Geometry check sheet. Reference: the model listing, model coordinates, mm. Face numbers are marked on the shaded views. A direction names the side the tool comes from. Give positions to 0.01 mm unless a question says otherwise; leave off trailing zeros. Write each loop counter-clockwise with the first axis right and the second up, starting at its lowest first coordinate (ties: lowest second). Pieces come first, ordered by that corner, then holes.
(1) Mould release check, pull along X, two halves, no side actions. Record for the marked faces 1, 2, 3 and 4: +X half, -X half, draft (parallel to the pull), parting line (faces both ways), or undercut.
(2) Thickness scan on line 1 along X through (y, z) = (-12, 5) (3 decimals); line 2 along X through (y, z) = (-8, 14.5) (3 decimals); line 3 along Y through (x, z) = (35, 32). Record the ranges inside material, lowest first.
(3) Cross-section at A-A (y = -21). Record the boundary of the cut face in (x, z) (3 decimals).
(4) Cross-section at B-B (y = 11.5). Record the boundary of the cut face in (x, z) (3 decimals).
(5) Depth check by flat-ended pin: P1, Ø16.5, axis at x = 2, y = 47, coming from the +Z side (3 decimals); P2, Ø2.5, axis at x = 59.5, y = 0, coming from the -Z side; P3, Ø8.5, axis at y = 13, z = 20.5, coming from the -X side (3 decimals). Enter the tip coordinate at first touch or a pass-through.
(6) Cross-section at C-C (y = 38.5). Record the boundary of the cut face in (x, z) (3 decimals), and give its area (3 significant figures).
(7) Tool access check on the marked faces 5, 6 and 7. Record the directions out of +Z, -Z, +X, -X, +Y, -Y that give a thin tool (end or side, any length) a straight path to the whole face; none if there is none.
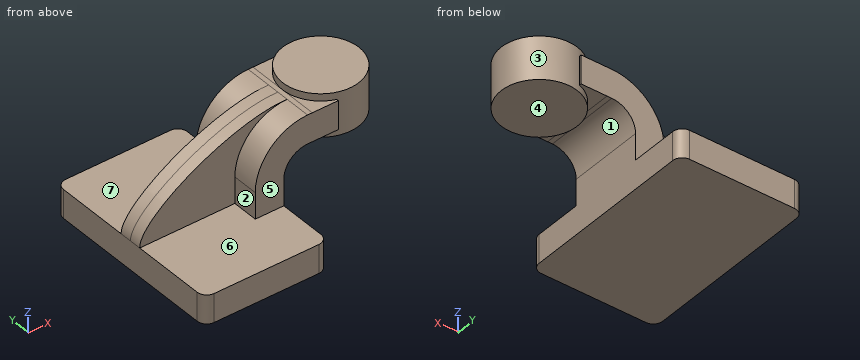
```python
from build123d import *

# Parameters (mm, degrees)
F1_DEPTH = 63.5
F2_DEPTH = 25.4
F3_DEPTH = 7.9375
F0_W     = 25.4
F0_H     = 28.575
F5_R     = 6.35


with BuildPart() as f1:
    # F0 (on Front) → F1 (new body, symmetric)
    with BuildSketch(Plane.XZ):
        Polygon((22.225, 9.525), (-41.275, 9.525), (-41.275, -9.525), (41.275, -9.525), (41.275, 9.525), align=None)
    extrude(amount=F1_DEPTH, both=True)

    # F0 (on Front) → F2 (join, symmetric)
    with BuildSketch(Plane.XZ):
        with BuildLine():
            Line((22.225, 27.000148), (22.225, 9.525))
            Line((22.225, 9.525), (41.275, 9.525))
            Line((41.275, 9.525), (41.275, 27.000148))
            ThreePointArc((41.275, 27.000148), (45.924666, 38.225454), (57.14996, 42.875148))
            Line((57.14996, 42.875148), (60.325, 42.875156))
            Line((60.325, 42.875156), (60.325, 61.925156))
            Line((60.325, 61.925156), (57.149911, 61.925148))
            ThreePointArc((57.149911, 61.925148), (32.454264, 51.695821), (22.225, 27.000148))
        make_face()
        Polygon((77.666241, 61.9252), (60.325, 61.925156), (60.325, 42.875156), (77.66629, 42.8752), align=None)
    extrude(amount=F2_DEPTH, both=True)

    # F0 (on Front) → F3 (join, symmetric)
    with BuildSketch(Plane.XZ):
        with BuildLine():
            add(Edge.make_bspline(
                [(-41.275, 9.525), (-41.347746, 28.786404), (20.412168, 63.539438), (57.149911, 61.925148)],
                knots=[0, 0, 0, 0, 111.504433, 111.504433, 111.504433, 111.504433], degree=3))
            Line((-41.275, 9.525), (22.225, 9.525))
            Line((22.225, 9.525), (22.225, 27.000148))
            ThreePointArc((22.225, 27.000148), (32.454264, 51.695821), (57.149911, 61.925148))
        make_face()
    extrude(amount=F3_DEPTH, both=True)

    # F0 (on Front) → F4 (revolve)
    with BuildSketch(Plane.XZ):
        with Locations((98.425, 52.3875)):
            Rectangle(F0_W, F0_H)
    revolve(axis=Axis((85.725, 0, 52.3875), (0, 0, -1)))

    # F5
    f5_edges = [f1.edges().sort_by_distance(p)[0] for p in [
        (41.275, -63.5, 0),
        (-41.275, -63.5, 0),
        (41.275, 63.5, 0),
        (-41.275, 63.5, 0),
    ]]
    fillet(f5_edges, radius=F5_R)


solid = f1.part
```
Reply:
1. face 1: undercut
1. face 2: -X half
1. face 3: undercut
1. face 4: draft
2. line 1: x = -41.275 to 41.275
2. line 2: x = 22.225 to 41.275
2. line 3: y = -25.4 to 25.4
3. outline: (-41.275, -9.525) - (41.275, -9.525) - (41.275, 27) arc R15.875 cw to (57.15, 42.875) - (71.437, 42.875) - (71.437, 38.1) - (100.013, 38.1) - (100.013, 66.675) - (71.437, 66.675) - (71.437, 61.925) - (57.15, 61.925) arc R34.925 ccw to (22.225, 27) - (22.225, 9.525) - (-41.275, 9.525) - close
4. outline: (-41.275, -9.525) - (41.275, -9.525) - (41.275, 27) arc R15.875 cw to (57.15, 42.875) - (63.077, 42.875) - (63.077, 38.1) - (108.373, 38.1) - (108.373, 66.675) - (63.077, 66.675) - (63.077, 61.925) - (57.15, 61.925) arc R34.925 ccw to (22.225, 27) - (22.225, 9.525) - (-41.275, 9.525) - close
5. P1: stops at z = 9.525
5. P2: stops at z = 38.1
5. P3: stops at x = 22.225
6. outline: (-41.275, -9.525) - (41.275, -9.525) - (41.275, 9.525) - (-41.275, 9.525) - close
6. area: 1,570 mm2
7. face 5: +Z, +X, -X, -Y
7. face 6: +Z, -X, -Y
7. face 7: +Z, -X, +Y
